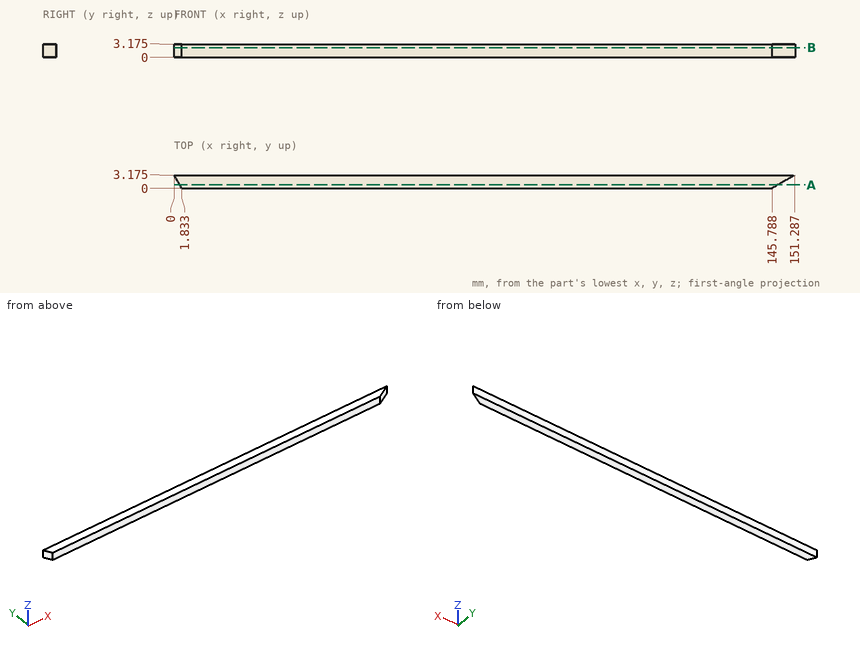
Could you check a few things on this drawing? It's one solid part, dimensions in mm from its lowest x, y, z. Round coordinates to 2 decimals unless told otherwise and drop trailing zeros. Write each loop counter-clockwise with the first axis right and the second up, starting at its lowest first coordinate (ties: lowest second). Pieces come first, ordered by that corner, then holes. Notation, with made-up numbers: (80.25, -22.75) -> (136.25, -22.75) arc R13 ccw to (136.25, -17.75) -> close; hole circle Ø3 at (23.5, 26.25). An arc over 180 degrees is marked (long way). One line per item, written item: value.
1) Suppose I cut it at A-A on y = 0.75. List the corners of the cut face in (x, z) for me (3 decimals).
Filled sheet:
outline: (1.4, 0) -> (147.087, 0) -> (147.087, 3.175) -> (1.4, 3.175) -> close
2) Suppose I cut it at B-B on z = 2.3. List the corners of the cut face in (x, y) for me (1 decimal).
Filled sheet:
outline: (0, 3.2) -> (1.8, 0) -> (145.8, 0) -> (151.3, 3.2) -> close
3) I'm going to push flat-ended pins straight in: pin 1 Ø1 at (y, z) = (2.5, 2.5) entering from -X; pin 2 Ø1.5 at (y, z) = (0.5, 2.5) entering from +X. Where does each tip first touch, or does it pass through?
Filled sheet:
pin 1: stops at x = 0.1
pin 2: stops at x = 147.95
4) If I drill on line 1 (X direction, y = 1.8, z = 0.45) (1 decimal); line 2 (X direction, y = 2.65, z = 0.7), over which ranges is the centre line in solid material (lowest first)? Write a range as [from, to].
Filled sheet:
line 1: x = [0.8, 148.9]
line 2: x = [0.3, 150.38]
